The model under review builds one solid part; all positions refer to its coordinate system, in mm. A direction names the side the tool comes from. Round coordinates to 2 decimals unless told otherwise and drop trailing zeros. Write each loop counter-clockwise with the first axis right and the second up, starting at its lowest first coordinate (ties: lowest second). Pieces come first, ordered by that corner, then holes. Notation, with made-up numbers: (42.25, 4.5) - (60.25, 4.5) arc R19 cw to (60.25, 11.5) - close; hole circle Ø8 at (63.25, 37). An arc over 180 degrees is marked (long way). One line per question, with ' | ' between items. Start each with the question number.
Autodesk Inventor part; units mm, degrees
ref_plane "YZ Plane" through (0, 0, 0) normal (1, 0, 0) x (0, 1, 0)
ref_plane "XZ Plane" through (0, 0, 0) normal (0, 1, 0) x (-1, 0, 0)
ref_plane "XY Plane" through (0, 0, 0) normal (0, 0, 1) x (1, 0, 0)
sketch "Sketch1" plane through (0, 0, 0) normal (0, 1, 0) x (-1, 0, 0)
  line L0 (0, 0) -> (0, -12.5)
  line L1 (0, -12.5) -> (20, -12.5)
  line L2 (20, -12.5) -> (20, -15.5)
  line L3 (20, -15.5) -> (0, -15.5)
  line L4 (0, -15.5) -> (0, -12.5)
  line L5 (0, 0) -> (0, 3)
  line L6 (0, 3) -> (20, 3)
  line L7 (20, 3) -> (20, 0)
  line L8 (20, 0) -> (0, 0)
  line L9 (20, 0) -> (20, -12.5)
  line L10 (20, -6.25) -> (30, -6.25)
  line L11 (30, -6.25) -> (40, -6.25)
  line L12 (40, -6.25) -> (40, 23.75)
  line L13 (20, -6.25) -> (20, 23.75)
  line L14 (20, 23.75) -> (22, 23.75)
  line L15 (40, 23.75) -> (38, 23.75)
  line L16 (29, 13.75) -> (22, 23.75)
  line L17 (31, 13.75) -> (38, 23.75)
  line L18 (31, 13.75) -> (31, -6.25)
  line L19 (29, 13.75) -> (29, -6.25)
  line L20 (20, -15.5) -> (27, -15.5)
  line L21 (27, -15.5) -> (40, -6.25)
  line L22 (20, 3) -> (12, 3)
  line L23 (20, 3) -> (20, 11)
  line L24 (20, 11) -> (12, 3)
  line L25 (20, 3) -> (12, 3)
  line L26 (20, 3) -> (20, 11)
  dimension "d0" = 12.5
  dimension "d1" = 20
  dimension "d2" = 3
  dimension "d3" = 3
  dimension "d4" = 20
  dimension "d5" = 10
  dimension "d6" = 10
  dimension "d7" = 30
  dimension "d8" = 2
  dimension "d9" = 2
  dimension "d13" = 7
  dimension "d22" = 8
  dimension "d23" = 8
extrude "Extrusion1" add sketch "Sketch1" along normal blind 14.5 contours L5 L6 L7 L8 | L1 L2 L3 L4
extrude "Extrusion2" add sketch "Sketch1" along normal blind 4 contours L8 L9 L1 L0 | L9 L10 L11 L21 L20 L2
extrude "Extrusion3" add sketch "Sketch1" along normal blind 7 contours L7 L13 L14 L16 L19 L10 L9 | L11 L18 L17 L15 L12
sketch "Sketch2" plane through (-40, 0, -6.25) normal (-1, 0, 0) x (0, 0, 1)
  line L0 (6.25, 4) -> (-6.25, 4)
  line L1 (0, 4) -> (30, 7)
  line L2 (30, 7) -> (30, 0)
  line L3 (30, 0) -> (30, 7)
  line L4 (30, 0) -> (0, 0)
  line L5 (9.25, 0) -> (-9.25, 0)
  line L6 (0, 4) -> (0, 0)
  line L7 (0, 0) -> (0, 4)
  line L8 (0, 0) -> (0, 4)
  line L9 (0, 4) -> (0, 7)
  line L10 (0, 4) -> (0, 7)
  line L11 (0, 7) -> (30, 7)
  point P0 (6.25, 0)
extrude "Extrusion5" add sketch "Sketch1" along normal blind 4 contours L24 L13 L6
extrude "Extrusion6" cut sketch "Sketch2" against normal blind 20 contours L9 L11 L1
sketch "Sketch3" plane through (0, 14.5, -15.5) normal (0, 0, -1) x (-1, 0, 0)
  line L0 (20, 0) -> (0, 0)
  line L1 (0, 0) -> (20, 0)
  line L2 (10, 0) -> (20, 0)
  line L3 (15, 0) -> (15, -10.5)
  line L4 (20, -10.5) -> (12, -10.5)
  line L5 (15, -10.5) -> (15, -4.25)
  line L6 (10, 0) -> (0, 0)
  line L7 (5, 0) -> (5, -10.5)
  line L8 (0, -10.5) -> (20, -10.5)
  line L9 (5, -10.5) -> (5, -4.25)
  circle A0 centre (15, -4.25) radius 1.6
  circle A1 centre (5, -4.25) radius 1.6
  point P0 (0, -14.5)
  dimension "d28" = 6.25
  dimension "d29" = 6.25
  dimension "d30" = 3.2
  dimension "d31" = 3.2
extrude "Extrusion7" cut sketch "Sketch3" against normal blind 20 contours A0 L3 | L3 A0 | A1 L7 | L7 A1
fillet "Fillet1" radius 17 4 edges at (-31, 3, 13.75) (-29, 3, 13.75) (-27, 2, -15.5) (-40, 2, -6.25)
fillet "Fillet2" radius 5 2 edges at (-38, 3.5, 23.75) (-22, 3.5, 23.75)
properties part number "clip"
1. Clearance check with flat-ended pins moving along their axes: P1, Ø3, axis at x = -8, y = 7.5, coming from the +Z side; P2, Ø1, axis at x = -32.5, y = 6.5, coming from the +Z side; P3, Ø0.6, axis at x = -29.5, y = 1, coming from the +Z side; P4, Ø3.5, axis at x = -5, y = 10.25, coming from the -Z side. State where each tip first meets the part, or that it passes through.
2. Add section D-D, the plane z = 5. Write out the cut boundary in (x, y) (3 decimals), then the cut area to 3 significant figures.
3. Add section B-B, the plane y = 10.25. Write out the cut boundary in (x, z).
4. Add section A-A, the plane x = -15. Write out the cut boundary in (y, z).
5. Wall thickness on line 1 along X through (y, z) = (10.25, -14.9); line 2 along Z through (x, y) = (-15.5, 12.25); line 3 along Y through (x, z) = (-5, -14): over which ranges is each line inside the solid? List them lowest first. Write a range as [from, to].
6. Machinability: for faces 1 (the face through (-20, 10, 1)), 2 (the face through (-10, 7, 3)), 3 (the face through (-10, 9, 0)), 4 (the face through (-10, 9, -12.5)), 5 (the face through (-31.81, 3.26, 13.57)), which of the approach directions +Z, -Z, +X, -X, +Y, -Y give a long, thin tool a straight path to every point of the face, cutting with its end or side? Answer none if there is none.
7. Add section C-C, the plane y = 7.5. Write out the cut boundary in (x, z), then the cut area to 3 significant figures.
8. The part is to be moulded in two halves that separate along Y. For faces 6 (the face through (-20, 9, -14)), 7 (the face through (-10, 14.5, -14)), 8 (the face through (-13.4, 10.3, 1.5)), say which applies: pulls with the +Y half, pulls with the -Y half, needs draft (parallel to the pull), parting line crosses it, or undercut.
Geometry check:
1) P1: stops at z = 3 | P2: stops at z = 16.27 | P3: stops at z = -6.25 | P4: stops at z = -15.5
2) outline: (-40, 0) - (-31, 0) - (-31, 5.125) - (-40, 5.125) - close; (-29, 0) - (-14, 0) - (-14, 4) - (-20, 4) - (-20, 5.125) - (-29, 5.125) - close | area: 116 mm2
3) outline: (-20, -15.5) - (-16.6, -15.5) - (-16.6, -12.5) - (-20, -12.5) - close; (-20, 0) - (-16.6, 0) - (-16.6, 3) - (-20, 3) - close; (-13.4, -15.5) - (-6.6, -15.5) - (-6.6, -12.5) - (-13.4, -12.5) - close; (-13.4, 0) - (-6.6, 0) - (-6.6, 3) - (-13.4, 3) - close; (-3.4, -15.5) - (0, -15.5) - (0, -12.5) - (-3.4, -12.5) - close; (-3.4, 0) - (0, 0) - (0, 3) - (-3.4, 3) - close
4) outline: (0, -15.5) - (8.65, -15.5) - (8.65, -12.5) - (4, -12.5) - (4, 0) - (8.65, 0) - (8.65, 3) - (4, 3) - (4, 6) - (0, 6) - close; (11.85, -15.5) - (14.5, -15.5) - (14.5, -12.5) - (11.85, -12.5) - close; (11.85, 0) - (14.5, 0) - (14.5, 3) - (11.85, 3) - close
5) line 1: x = [-20, -16.6], [-13.4, -6.6], [-3.4, 0] | line 2: z = [-15.5, -12.5], [0, 3] | line 3: y = [0, 8.65], [11.85, 14.5]
6) face 1: -Z, -X, +Y | face 2: +Z, +X, +Y | face 3: +X, +Y | face 4: +X, -X, +Y | face 5: +Z, +Y, -Y
7) outline: (-20, -15.5) - (0, -15.5) - (0, -12.5) - (-20, -12.5) - close; (-20, 0) - (0, 0) - (0, 3) - (-20, 3) - close | area: 120 mm2
8) face 6: needs draft | face 7: pulls with the +Y half | face 8: undercut
